For this review, take the finished solid that the model builds, in its own axes (mm). Face numbers are marked on the shaded views. A direction names the side the tool comes from. Give positions to 0.01 mm unless a question says otherwise; leave off trailing zeros. Order: outer loops, then holes, each group sorted by start corner. A loop starts at its lowest first (then second) coordinate and runs counter-clockwise, first axis right, second up. Notation, with made-up numbers: M -20,20.25 L -3,20.25 A11 cw -3,34.25 Z; hole C 45.5,30 d2. An arc over 180 degrees is marked long. Answer as CSV lines item,"result". Start each with the question number.
1. We need section B-B, the plane x = 13. Give the boundary of the cut face in (y, z).
2. For line 1 along Y through (x, z) = (13, -1.9); line 2 along Y through (x, z) = (13, 0.1); line 3 along Z through (x, y) = (2, 38.5), list the stretches that pass through material, from the lowest coordinate up.
3. Mouldability with a two-part tool opening along Y and no side actions: class the marked faces 3, 4 and 5 as pulls with the +Y half, pulls with the -Y half, needs draft (parallel to the pull), parting line crosses it, or undercut.
4. Machinability: for the marked faces 1 and 2, which of the approach directions +Z, -Z, +X, -X, +Y, -Y give a long, thin tool a straight path to every point of the face, cutting with its end or side? Answer none if there is none.
5. We need section D-D, the plane y = 6. Give the boundary of the cut face in (x, z), and give its area (3 significant figures).
6. We need section A-A, the plane y = 22.5. Give the boundary of the cut face in (x, z), and give its area (3 significant figures).
7. Clearance check with flat-ended pins moving along their axes: P1, Ø1.5, axis at x = 11, z = -1, coming from the +Y side; P2, Ø0.9, axis at y = 26, z = -1.5, coming from the -X side. State where each tip first meets the part, or that it passes through.
8. We need section C-C, the plane z = -2.5. Give the boundary of the cut face in (x, y).
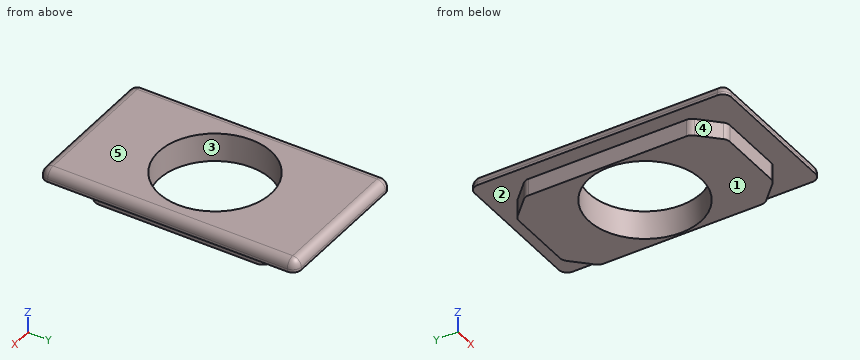
Autodesk Fusion 360 part; units mm, degrees
sketch "Sketch1" plane through (0, 0, 0) normal (0, 0, 1) x (1, 0, 0)
  line L0 (0, 0) -> (26, 0)
  line L1 (26, 0) -> (26, 45)
  line L2 (26, 45) -> (0, 45)
  line L3 (0, 45) -> (0, 0)
  line L4 (0, 45) -> (26, 0) construction
  circle A0 centre (13, 22.5) radius 9.85
  line L5 (6.75, 4) -> (19.25, 4)
  line L6 (23.25, 8) -> (23.25, 37)
  line L7 (19.25, 41) -> (6.75, 41)
  line L8 (2.75, 37) -> (2.75, 8)
  line L9 (6.75, 41) -> (2.75, 37)
  line L10 (23.25, 37) -> (19.25, 41)
  line L11 (6.75, 4) -> (2.75, 8)
  line L12 (23.25, 8) -> (19.25, 4)
  point P0 (2.75, 4)
  point P1 (23.25, 4)
  point P2 (23.25, 41)
  point P3 (2.75, 41)
  dimension "d1" = 19.7
  dimension "d2" = 26
  dimension "d3" = 45
  dimension "d4" = 20.5
  dimension "d5" = 2.75
  dimension "d6" = 4
  dimension "d7" = 37
  dimension "d8" = 4
  dimension "d9" = 4
  dimension "d10" = 4
  dimension "d11" = 4
  dimension "d12" = 4
  dimension "d13" = 4
  dimension "d14" = 4
  dimension "d15" = 4
extrude "Extrude1" add sketch "Sketch1" along normal blind 2 contours L0 L1 L2 L3 | L5 L6 L7 L8 L9 L10 L11 L12
extrude "Extrude2" add sketch "Sketch1" against normal blind 3 contours L5 L6 L7 L8 L9 L10 L11 L12
fillet "Fillet1" radius 1.5 16 edges at (26, 0, 1) (0, 0, 1) (0, 45, 1) (26, 45, 1) (6.75, 41, -1.5) (2.75, 37, -1.5) (19.25, 41, -1.5) (23.25, 37, -1.5) (23.25, 8, -1.5) (19.25, 4, -1.5) (6.75, 4, -1.5) (2.75, 8, -1.5) (13, 45, 2) (0, 22.5, 2) (13, 0, 2) (26, 22.5, 2)
equation "d5 = ( d2 - d4 ) / 2"
equation "d6 = ( d3 - d7 ) / 2"
equation "d9 = d8"
equation "d10 = d8"
equation "d11 = d10"
equation "d12 = d8"
equation "d13 = d12"
equation "d14 = d8"
equation "d15 = d14"
Result set:
1,outline,"M 0,0 L 4,0 L 4,-3 L 12.65,-3 L 12.65,2 L 1.5,2 A1.5 ccw 0,0.5 Z; M 32.35,-3 L 41,-3 L 41,0 L 45,0 L 45,0.5 A1.5 ccw 43.5,2 L 32.35,2 Z"
2,line 1,"4 to 12.65, 32.35 to 41"
2,line 2,"0 to 12.65, 32.35 to 45"
2,line 3,"0 to 2"
3,face 3,"undercut"
3,face 4,"pulls with the -Y half"
3,face 5,"needs draft"
4,face 1,"-Z, +X, -X, +Y, -Y"
4,face 2,"-Z"
5,outline,"M 0,0 L 4.75,0 L 4.75,-3 L 21.25,-3 L 21.25,0 L 26,0 L 26,0.5 A1.5 ccw 24.5,2 L 1.5,2 A1.5 ccw 0,0.5 Z"
5,area,"101 mm2"
6,outline,"M 0,0 L 2.75,0 L 2.75,-3 L 3.15,-3 L 3.15,2 L 1.5,2 A1.5 ccw 0,0.5 Z; M 22.85,-3 L 23.25,-3 L 23.25,0 L 26,0 L 26,0.5 A1.5 ccw 24.5,2 L 22.85,2 Z"
6,area,"14.0 mm2"
7,P1,"y = 41"
7,P2,"x = 2.75"
8,outline,"M 2.75,8.62 A1.5 ccw 3.19,7.56 L 6.31,4.44 A1.5 ccw 7.37,4 L 18.63,4 A1.5 ccw 19.69,4.44 L 22.81,7.56 A1.5 ccw 23.25,8.62 L 23.25,36.38 A1.5 ccw 22.81,37.44 L 19.69,40.56 A1.5 ccw 18.63,41 L 7.37,41 A1.5 ccw 6.31,40.56 L 3.19,37.44 A1.5 ccw 2.75,36.38 Z; hole C 13,22.5 d19.7"
